Read the model definition and answer for the solid it produces. Units are mm, in the model's axes. Give positions to 0.01 mm unless a question says otherwise; leave off trailing zeros. Loops run counter-clockwise (first coordinate to the right, second up) from the corner with the lowest first, then second, coordinate; pieces in that order, holes last. Notation, with made-up numbers: (35, 23.5) - (42, 23.5) arc R18 ccw to (42, 36.5) - close; hole circle Ø10 at (73, 70). An arc over 180 degrees is marked (long way). Put each result on its own line as item: value. Start each with the question number.
1. For a pull along Z with two mould halves and no side action, classify faces 1 (the flat face through (0, 6, -31.75)), 2 (the cylindrical face through (-0.05, 6.44, 1.23)), 3 (the flat face through (-1.32, 0, 0.44)) as released by +Z, released by -Z, zero draft, split by the parting line, or undercut.
2. A cutting plane is placed at A-A, the plane x = 0. Count the separate pieces of the cut face and the enclosed holes in it, plus the area to 3 significant figures.
3. A cutting plane is placed at B-B, the plane z = 0. Determine the outline of the cut face in (x, y), plus the area to 3 significant figures.
4. A cutting plane is placed at C-C, the plane y = 4.5. Determine the outline of the cut face in (x, z).
5. A cutting plane is placed at D-D, the plane x = 4. Determine the outline of the cut face in (y, z), plus the area to 3 significant figures.
6. Consider L1, parallel to Z at x = 0, y = 4; L2, parallel to Z at x = 2.5, y = 6.35; L3, parallel to X at y = 4, z = -12.7. Determine where each line is inside the solid, lowest interval first. Write a range as from..to.
Autodesk Inventor part; units mm, degrees
ref_plane "YZ Plane" through (0, 0, 0) normal (1, 0, 0) x (0, 1, 0)
ref_plane "XZ Plane" through (0, 0, 0) normal (0, 1, 0) x (-1, 0, 0)
ref_plane "XY Plane" through (0, 0, 0) normal (0, 0, 1) x (1, 0, 0)
sketch "Sketch1" plane through (0, 0, 0) normal (0, 1, 0) x (-1, 0, 0)
  line L0 (-6.35, -31.75) -> (6.35, -31.75)
  line L1 (6.35, -31.75) -> (6.35, 31.75)
  line L2 (6.35, 31.75) -> (-6.35, 31.75)
  line L3 (-6.35, 31.75) -> (-6.35, -31.75)
  line L4 (-6.35, -31.75) -> (6.35, 31.75) construction
  line L5 (6.35, -31.75) -> (-6.35, 31.75) construction
  point P0 (0, 0)
  dimension "d0" = 63.5
  dimension "d1" = 12.7
extrude "Extrusion1" add sketch "Sketch1" along normal blind 12.7
sketch "Sketch2" plane through (6.35, 0, 31.75) normal (1, 0, 0) x (0, 0, -1)
  line L0 (63.5, 0) -> (63.5, 12.7)
  line L1 (63.5, 6.35) -> (0, 6.35)
  line L2 (0, 0) -> (0, 12.7)
  line L3 (31.75, 6.35) -> (31.75, 12.7)
  point P0 (31.75, 0)
  point P1 (12.7, 6.35)
  point P2 (25.4, 6.35)
  point P3 (38.1, 6.35)
  point P4 (50.8, 6.35)
  dimension "d4" = 12.7
  dimension "d5" = 12.7
  dimension "d6" = 12.7
  dimension "d15" = 6.35
hole "Hole1" at (6.35, 6.35, 19.05) at (6.35, 6.35, 6.35) at (6.35, 6.35, -6.35) at (6.35, 6.35, -19.05) direction (-1, 0, 0) diameter 2.4638 end through all
sketch "Sketch3" plane through (0, 0, 0) normal (0, -1, 0) x (1, 0, 0)
  line L0 (6.35, 31.75) -> (6.35, -31.75)
  line L1 (6.35, 0) -> (-6.35, 0)
  line L2 (-6.35, -31.75) -> (-6.35, 31.75)
  point P0 (0, 0)
  point P1 (0, 25.4)
  point P2 (0, 12.7)
  point P3 (0, -12.7)
  point P4 (0, -25.4)
  point P5 (0, 0)
  dimension "d16" = 12.7
  dimension "d17" = 12.7
  dimension "d18" = 12.7
  dimension "d19" = 12.7
hole "Hole2" at (0, 0, 25.4) at (0, 0, 12.7) at (0, 0, -12.7) at (0, 0, -25.4) at (0, 0, 0) direction (0, 1, 0) diameter 2.4638 end through all
properties part number "Lead_Screw_Fixture_Side_Wall"
Return value:
1. face 1: released by -Z
1. face 2: undercut
1. face 3: zero draft
2. separate pieces: 6
2. enclosed holes: 4
2. area: 631 mm2
3. outline: (-6.35, 0) - (-1.23, 0) - (-1.23, 12.7) - (-6.35, 12.7) - close; (1.23, 0) - (6.35, 0) - (6.35, 12.7) - (1.23, 12.7) - close
3. area: 130 mm2
4. outline: (-6.35, -31.75) - (6.35, -31.75) - (6.35, 31.75) - (-6.35, 31.75) - close; hole circle Ø2.46 at (0, -25.4); hole circle Ø2.46 at (0, -12.7); hole circle Ø2.46 at (0, 0); hole circle Ø2.46 at (0, 12.7); hole circle Ø2.46 at (0, 25.4)
5. outline: (0, -31.75) - (12.7, -31.75) - (12.7, 31.75) - (0, 31.75) - close; hole circle Ø2.46 at (6.35, -19.05); hole circle Ø2.46 at (6.35, -6.35); hole circle Ø2.46 at (6.35, 6.35); hole circle Ø2.46 at (6.35, 19.05)
5. area: 787 mm2
6. L1: z = -31.75..-26.63, -24.17..-13.93, -11.47..-1.23, 1.23..11.47, 13.93..24.17, 26.63..31.75
6. L2: z = -31.75..-20.28, -17.82..-7.58, -5.12..5.12, 7.58..17.82, 20.28..31.75
6. L3: x = -6.35..-1.23, 1.23..6.35
